For this review, take the finished solid that the model builds, in its own axes (mm). Face numbers are marked on the shaded views. Give positions to 0.01 mm unless a question says otherwise; leave off trailing zeros. Loops run counter-clockwise (first coordinate to the right, second up) from the corner with the lowest first, then second, coordinate; pieces in that order, holes last. Notation, with made-up numbers: (80, 51) - (99, 51) arc R9 ccw to (99, 60) - close; hole circle Ø5 at (-21.75, 9). An arc over 180 degrees is marked (long way). Answer in a Markdown table with one row per item.
```python
from build123d import *

# Parameters (mm, degrees)
SKETCH1_W           = 8.5
SKETCH1_H           = 6.6
BOSS_EXTRUDE1_DEPTH = 4.2
CUT_EXTRUDE1_DEPTH  = 14.2
CHAMFER1_SIZE       = 1.073169072
CHAMFER1_SIZE_2     = 1
FILLET1_R           = 1
FILLET2_R           = 0.2
FILLET3_R           = 0.02
SKETCH3_R           = 0.5
CUT_EXTRUDE2_DEPTH  = 14.2
CHAMFER2_SIZE       = 0.1


with BuildPart() as part:
    # Sketch1 → Boss-Extrude1 (new body)
    with BuildSketch(Plane(origin=(0, 0, 0), x_dir=(1, 0, 0), z_dir=(0, 1, 0))):
        Rectangle(SKETCH1_W, SKETCH1_H)
    extrude(amount=BOSS_EXTRUDE1_DEPTH)

    # Sketch2 → Cut-Extrude1 (cut)
    with BuildSketch(Plane(origin=(4.25, 0, 0), x_dir=(0, 0, -1), z_dir=(1, 0, 0))):
        with BuildLine():
            Line((-3.3, 3.9), (-5.253535024, 5.241651662))
            Line((-5.253535024, 5.241651662), (3.889156526, 7.141243929))
            Line((3.889156526, 7.141243929), (5.679183493, 5.077233243))
            Line((5.679183493, 5.077233243), (3.3, 3.9))
            ThreePointArc((3.3, 3.9), (0, 4.009018851), (-3.3, 3.9))
        make_face()
        with BuildLine():
            Line((4.717394395, 0), (0, -2.904825783))
            Line((0, -2.904825783), (-4.70037365, 0))
            ThreePointArc((-4.70037365, 0), (0.008510373, 0.222229748), (4.717394395, 0))
        make_face()
    extrude(amount=-CUT_EXTRUDE1_DEPTH, mode=Mode.SUBTRACT)

    # Chamfer1
    # the kernel refuses this chamfer: 1.073169072, 1 mm, written as the material it takes off along each edge
    with BuildSketch(Plane(origin=(7.014554566, 3.9, -3.3), x_dir=(0, -1, 0), z_dir=(-1, 0, 0))) as chamfer1_piece_1:
        with BuildLine():
            Line((CHAMFER1_SIZE, 0), (-0.05556839, 0.98868238))
            ThreePointArc((-0.05556839, 0.98868238), (-0.031072564, 0.509202078), (0, 0))
            Line((0, 0), (CHAMFER1_SIZE, 0))
        make_face()
    extrude(amount=14.029109133, mode=Mode.SUBTRACT)
    with BuildSketch(Plane(origin=(6.981889399, 3.9, 3.3), x_dir=(0, 0.05541549441613883, -0.9984633808901632), z_dir=(-1, 0, 0))) as chamfer1_piece_2:
        with BuildLine():
            Line((1.060391539, 0), (-CHAMFER1_SIZE_2 * 0.0554154944161, CHAMFER1_SIZE_2 * 0.99846338089))
            Line((-CHAMFER1_SIZE_2 * 0.0554154944161, CHAMFER1_SIZE_2 * 0.99846338089), (0, 0))
            ThreePointArc((0, 0), (0.546186707, -0.002808597), (1.060391539, 0))
        make_face()
    extrude(amount=13.963778797, mode=Mode.SUBTRACT)

    # Fillet1
    fillet1_edges = [part.edges().sort_by_distance(p)[0] for p in [
        (0, 0.11377308, -3.3),
        (0, 0.112647256, 3.3),
    ]]
    fillet(fillet1_edges, radius=FILLET1_R)

    # Fillet2
    fillet2_edges = [part.edges().sort_by_distance(p)[0] for p in [
        (0, 2.826830928, -3.3),
        (0, 3.958762121, 2.241237879),
        (0, 3.95556839, -2.31131762),
        (0, 2.9, 3.3),
    ]]
    fillet(fillet2_edges, radius=FILLET2_R)

    # Fillet3
    fillet3_edges = [part.edges().sort_by_distance(p)[0] for p in [
        (4.25, 0.22222905, -0.000158372),
        (4.25, 0.447906277, -2.99103865),
        (4.25, 0.447022472, 2.990917901),
        (-4.25, 0.22222905, -0.000158372),
        (-4.25, 0.447906277, -2.99103865),
        (-4.25, 0.447022472, 2.990917901),
        (4.25, 1.961174313, -3.3),
        (-4.25, 1.961174313, -3.3),
        (4.25, 1.993556495, 3.3),
        (4.25, 3.387413237, -2.808975408),
        (4.25, 4.009009057, -0.031295116),
        (4.25, 3.431189943, 2.768810057),
        (4.25, 2.893693974, 3.284775907),
        (4.25, 3.94545632, 2.235294601),
        (4.25, 3.939907453, -2.30368815),
        (4.25, 2.822018564, -3.287202247),
        (-4.25, 3.387413237, -2.808975408),
        (-4.25, 1.993556495, 3.3),
        (-4.25, 3.431189943, 2.768810057),
        (-4.25, 4.009009057, -0.031295116),
        (-4.25, 2.893693974, 3.284775907),
        (-4.25, 3.94545632, 2.235294601),
        (-4.25, 3.939907453, -2.30368815),
        (-4.25, 2.822018564, -3.287202247),
    ]]
    fillet(fillet3_edges, radius=FILLET3_R)

    # Sketch3 → Cut-Extrude2 (cut)
    with BuildSketch(Plane.ZY.offset(4.25)):
        with Locations((-1.9, 1.5)):
            Circle(SKETCH3_R)
        with Locations((1.3, 1.5)):
            Circle(SKETCH3_R)
    extrude(amount=-CUT_EXTRUDE2_DEPTH, mode=Mode.SUBTRACT)

    # Chamfer2
    chamfer2_edges = [part.edges().sort_by_distance(p)[0] for p in [
        (4.25, 1.5, -2.4),
        (-4.25, 1.5, -2.4),
        (4.25, 1.5, 0.8),
        (-4.25, 1.5, 0.8),
    ]]
    chamfer(chamfer2_edges, length=CHAMFER2_SIZE)


solid = part.part
```
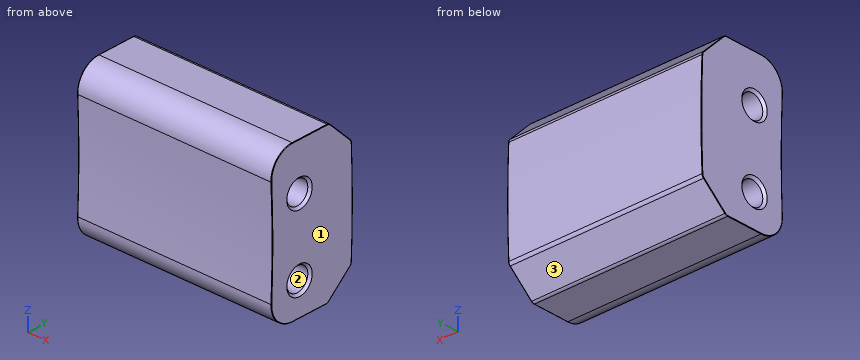
1. Wall thickness on line 1 (Y direction, x = -2, z = -0.5); line 2 (Y direction, x = 3.25, z = 1); line 3 (Y direction, x = 2.5, z = 1.3): over which ranges is each line inside the solid? List them lowest first. Write a range as [from, to].
Values:
| item | result |
|---|---|
| line 1 | y = [0.22, 4.01] |
| line 2 | y = [0.21, 1.1], [1.9, 4] |
| line 3 | y = [0.21, 1], [2, 3.99] |
2. Mouldability with a two-part tool opening along Z and no side actions: class the marked faces 1, 2 and 3 as released by +Z, released by -Z, zero draft, split by the parting line, or undercut.
Values:
| item | result |
|---|---|
| face 1 | zero draft |
| face 2 | undercut |
| face 3 | released by -Z |
3. We need section B-B, the plane x = -0.75. Give the boundary of the cut face in (y, z).
Values:
| item | result |
|---|---|
| outline | (0.17, -2.26) arc R1 ccw to (1.17, -3.3) - (2.75, -3.3) arc R0.2 ccw to (2.88, -3.25) - (3.89, -2.37) arc R0.2 ccw to (3.96, -2.23) arc R50 ccw to (3.96, 2.16) arc R0.2 ccw to (3.9, 2.3) - (2.96, 3.24) arc R0.2 ccw to (2.82, 3.3) - (1.17, 3.3) arc R1 ccw to (0.17, 2.25) arc R50 cw to start; hole circle Ø1 at (1.5, -1.9); hole circle Ø1 at (1.5, 1.3) |
4. We need section A-A, the plane y = 1.5. Count the separate pieces of the cut face and the enclosed holes in it, and give its area (3 significant figures).
Values:
| item | result |
|---|---|
| separate pieces | 3 |
| enclosed holes | 0 |
| area | 39.1 mm^2 |
